Read the model definition and answer for the solid it produces. Units are mm, in the model's axes. Face numbers are marked on the shaded views. Coordinates: 2 decimals unless noted, no trailing zeros. Write each loop counter-clockwise with the first axis right and the second up, starting at its lowest first coordinate (ties: lowest second). Pieces come first, ordered by that corner, then holes.
Item 1: Section A-A (z = -5) is taken. Give the vertices of the cut face in (x, y).
Item 2: Determine the mould class of the marked faces 1, 2 and 3 for opening direction X: released by +X, released by -X, zero draft, split by the parting line, or undercut.
Item 3: Straight lines are drawn through the part: probe 1 along Y at (x, z) = (38.1, -2.25); probe 2 along Y at (x, z) = (13, -5.75); probe 3 along X at (y, z) = (25.4, -7.9). For each, find the intervals that lie inside material, in ascending order.
Item 4: Each of these flat-tipped pins is pushed along its axis until it touches: P1, Ø3, axis at x = 12.7, y = 12.7, coming from the +Z side; P2, Ø1.5, axis at x = 12.5, z = -7.5, coming from the +Y side. Where does it stop, or does it pass through?
Item 5: Section C-C (x = 38.1) is taken. Give the vertices of the cut face in (y, z).
Item 6: Section B-B (y = 12.7) is taken. Give the vertices of the cut face in (x, z), then the cut area to 3 significant figures.
Item 7: Section D-D (y = 25.4) is taken. Give the vertices of the cut face in (x, z), then the cut area to 3 significant figures.
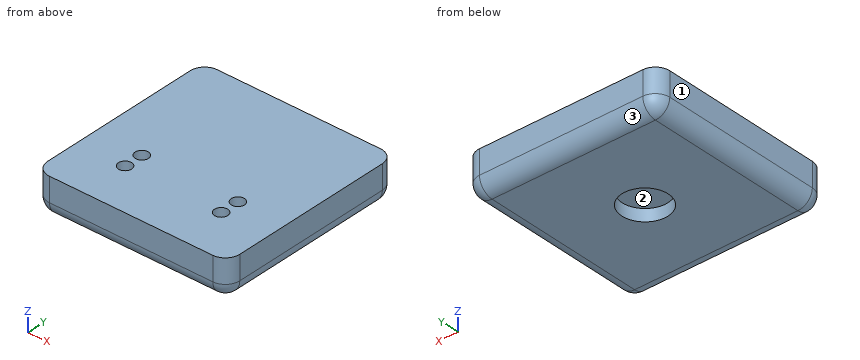
from build123d import *

# Parameters (mm, degrees)
F0_R     = 1.7526
F1_DEPTH = 10.16
F2_DEPTH = 7.62
F3_R     = 6.1
F4_DEPTH = 3.2
F5_R     = 3.81


with BuildPart() as f1:
    # F0 (on Top) → F1 (new body)
    with BuildSketch(Plane.XY):
        with BuildLine():
            ThreePointArc((0, 3.81), (1.1159231637, 1.1159231637), (3.81, 0))
            Line((3.81, 0), (46.99, 0))
            ThreePointArc((46.99, 0), (49.6840768363, 1.1159231637), (50.8, 3.81))
            Line((50.8, 3.81), (50.8, 46.99))
            ThreePointArc((50.8, 46.99), (49.6840768363, 49.6840768363), (46.99, 50.8))
            Line((46.99, 50.8), (3.81, 50.8))
            ThreePointArc((3.81, 50.8), (1.1159231637, 49.6840768363), (0, 46.99))
            Line((0, 46.99), (0, 3.81))
        make_face()
        with Locations((12.7, 12.7)):
            Circle(F0_R, mode=Mode.SUBTRACT)
        with Locations((12.7, 17.78)):
            Circle(F0_R, mode=Mode.SUBTRACT)
        with Locations((38.1, 12.7)):
            Circle(F0_R, mode=Mode.SUBTRACT)
        with Locations((38.1, 17.78)):
            Circle(F0_R, mode=Mode.SUBTRACT)
        with Locations((12.7, 17.78)):
            Circle(F0_R)
        with Locations((38.1, 17.78)):
            Circle(F0_R)
        with Locations((12.7, 12.7)):
            Circle(F0_R)
        with Locations((38.1, 12.7)):
            Circle(F0_R)
    extrude(amount=-F1_DEPTH)

    # F0 (on Top) → F2 (cut)
    with BuildSketch(Plane.XY):
        with Locations((12.7, 17.78)):
            Circle(F0_R)
        with Locations((38.1, 17.78)):
            Circle(F0_R)
        with Locations((38.1, 12.7)):
            Circle(F0_R)
        with Locations((12.7, 12.7)):
            Circle(F0_R)
    extrude(amount=-F2_DEPTH, mode=Mode.SUBTRACT)

    # F3 (on face) → F4 (cut)
    with BuildSketch(Plane(origin=(0, 0, -10.16), x_dir=(1, 0, 0), z_dir=(0, 0, -1))):
        with Locations((25.4, -25.4)):
            Circle(F3_R)
    extrude(amount=-F4_DEPTH, mode=Mode.SUBTRACT)

    # F5
    f5_edges = [f1.edges().sort_by_distance(p)[0] for p in [
        (25.4, 0, -10.16),
    ]]
    fillet(f5_edges, radius=F5_R)


solid = f1.part
Established:
1. outline: (0, 3.81) arc R3.81 ccw to (3.81, 0) - (46.99, 0) arc R3.81 ccw to (50.8, 3.81) - (50.8, 46.99) arc R3.81 ccw to (46.99, 50.8) - (3.81, 50.8) arc R3.81 ccw to (0, 46.99) - close; hole circle Ø3.51 at (12.7, 12.7); hole circle Ø3.51 at (12.7, 17.78); hole circle Ø3.51 at (38.1, 12.7); hole circle Ø3.51 at (38.1, 17.78)
2. face 1: released by -X
2. face 2: undercut
2. face 3: zero draft
3. probe 1: y = 0 to 10.95, 14.45 to 16.03, 19.53 to 50.8
3. probe 2: y = 0 to 10.97, 14.43 to 16.05, 19.51 to 50.8
3. probe 3: x = 0.33 to 19.3, 31.5 to 50.47
4. P1: stops at z = -7.62
4. P2: stops at y = 50.78
5. outline: (0, -6.35) arc R3.81 ccw to (3.81, -10.16) - (46.99, -10.16) arc R3.81 ccw to (50.8, -6.35) - (50.8, 0) - (19.53, 0) - (19.53, -7.62) - (16.03, -7.62) - (16.03, 0) - (14.45, 0) - (14.45, -7.62) - (10.95, -7.62) - (10.95, 0) - (0, 0) - close
6. outline: (0, -6.35) arc R3.81 ccw to (3.81, -10.16) - (46.99, -10.16) arc R3.81 ccw to (50.8, -6.35) - (50.8, 0) - (39.85, 0) - (39.85, -7.62) - (36.35, -7.62) - (36.35, 0) - (14.45, 0) - (14.45, -7.62) - (10.95, -7.62) - (10.95, 0) - (0, 0) - close
6. area: 456 mm2
7. outline: (0, -6.35) arc R3.81 ccw to (3.81, -10.16) - (19.3, -10.16) - (19.3, -6.96) - (31.5, -6.96) - (31.5, -10.16) - (46.99, -10.16) arc R3.81 ccw to (50.8, -6.35) - (50.8, 0) - (0, 0) - close
7. area: 471 mm2
